Geometry check sheet. Reference: the model listing, model coordinates, mm. A direction names the side the tool comes from. Round coordinates to 2 decimals unless told otherwise and drop trailing zeros. Loops run counter-clockwise (first coordinate to the right, second up) from the corner with the lowest first, then second, coordinate; pieces in that order, holes last. Notation, with made-up numbers: M 18.5,81.5 L 48.5,81.5 A31 cw 48.5,110.5 Z; hole C 59,-25 d9. An arc over 180 degrees is marked long. Use one line per item in the form item = value. Start each with the question number.
1. Go/stop test with flat-tipped pins: pin 1 (4 mm diameter, centred on y = -23.79, z = 7.45, fed in from +X); pin 2 (4 mm diameter, centred on x = 9.5, z = 4, fed in from -Y); pin 3 (2.5 mm diameter, centred on x = 7, z = 5.5, fed in from +Y). Record where each tip stops, or that it passes through.
2. Cross-section at D-D (x = -14.5). Record the boundary of the cut face in (y, z), then the cut area to 3 significant figures.
3. Cross-section at C-C (y = -14). Record the boundary of the cut face in (x, z).
4. Material ranges on line 1 (Y direction, x = -41.95, z = 7.45); line 2 (Y direction, x = -34, z = 9); line 3 (Y direction, x = -39.55, z = 7.45), recorded low to high.
5. Cross-section at B-B (z = 7.45). State how many separate pieces and enclosed holes the cut face has, then the cut area to 3 significant figures.
6. Set-up check for faces 4 (the flat face through (10.19, 5, 6)), 5 (the cylindrical face through (-40.73, -20.62, 7.03)), 6 (the cylindrical face through (9.75, -7.07, 5.92)): record each of +Z, -Z, +X, -X, +Y, -Y from which the full face is reachable in a straight line by a thin tool's end or side.
7. Cross-section at A-A (y = 0). Record the boundary of the cut face in (x, z).
8. Draft check along Y on faces 1 (the cylindrical face through (-41.796, -35.377, 6.084)), 2 (the flat face through (7.28, 5.25, 5.92)), 3 (the flat face through (-5, -10.19, 6)). Enter one of: pulls with the +Y half, pulls with the -Y half, needs draft (parallel to the pull), parting line crosses it, or undercut.
```python
from build123d import *

# Parameters (mm, degrees)
BOSS_EXTRUDE1_DEPTH = 12
FILLET1_R           = 5
FILLET2_R           = 5
CUT_EXTRUDE1_REACH  = 74.499
SKETCH3_R           = 3.2
CHAMFER1_SIZE       = 0.2


with BuildPart() as part:
    # Sketch2 → Boss-Extrude1 (new body)
    with BuildSketch(Plane.XY):
        with BuildLine():
            Line((-10.5918, -13), (-5.317126718, -13))
            Line((-5.317126718, -13), (-4.287512407, -13))
            ThreePointArc((-4.287512407, -13), (-3.333616586, -12.604883414), (-2.9385, -11.650987593))
            Line((-2.9385, -11.650987593), (-2.9385, -11.539212407))
            ThreePointArc((-2.9385, -11.539212407), (-3.333616586, -10.585316586), (-4.287512407, -10.1902))
            Line((-4.287512407, -10.1902), (-6.416408329, -10.1902))
            ThreePointArc((-6.416408329, -10.1902), (-7.137514675, -9.708134418), (-6.967711912, -8.857517813))
            Line((-6.967711912, -8.857517813), (-3.740331666, -5.636015806))
            ThreePointArc((-3.740331666, -5.636015806), (-2.808257752, -5.01414519), (-1.709253557, -4.7958))
            Line((-1.709253557, -4.7958), (1.709253557, -4.7958))
            ThreePointArc((1.709253557, -4.7958), (2.808257752, -5.01414519), (3.740331666, -5.636015806))
            Line((3.740331666, -5.636015806), (6.967711912, -8.857517813))
            ThreePointArc((6.967711912, -8.857517813), (7.137514675, -9.708134418), (6.416408329, -10.1902))
            Line((6.416408329, -10.1902), (4.287512407, -10.1902))
            ThreePointArc((4.287512407, -10.1902), (3.333616586, -10.585316586), (2.9385, -11.539212407))
            Line((2.9385, -11.539212407), (2.9385, -11.650987593))
            ThreePointArc((2.9385, -11.650987593), (3.333616586, -12.604883414), (4.287512407, -13))
            Line((4.287512407, -13), (5.317126718, -13))
            Line((5.317126718, -13), (9.550465633, -13))
            Line((9.550465633, -13), (10.564722121, -12.999847763))
            ThreePointArc((10.564722121, -12.999847763), (12.294654751, -12.29465435), (12.999847757, -10.564721553))
            Line((12.999847757, -10.564721553), (13, -9.550422515))
            Line((13, -9.550422515), (13, -6.3330836))
            Line((13, -6.3330836), (13, -5.3170836))
            Line((13, -5.3170836), (13, -4.287469289))
            ThreePointArc((13, -4.287469289), (12.604883414, -3.333573468), (11.650987593, -2.938456882))
            Line((11.650987593, -2.938456882), (11.539212407, -2.938456882))
            ThreePointArc((11.539212407, -2.938456882), (10.585316586, -3.333573468), (10.1902, -4.287469289))
            Line((10.1902, -4.287469289), (10.1902, -6.402089023))
            ThreePointArc((10.1902, -6.402089023), (9.74154152, -7.073969797), (8.94902056, -6.917034355))
            Line((8.94902056, -6.917034355), (5.652895046, -3.628441884))
            ThreePointArc((5.652895046, -3.628441884), (5.027976112, -2.694919539), (4.8085, -1.593185507))
            Line((4.8085, -1.593185507), (4.8085, 1.593185507))
            ThreePointArc((4.8085, 1.593185507), (5.027976112, 2.694919539), (5.652895046, 3.628441884))
            Line((5.652895046, 3.628441884), (8.94902056, 6.917034355))
            ThreePointArc((8.94902056, 6.917034355), (9.74154152, 7.073969797), (10.1902, 6.402089023))
            Line((10.1902, 6.402089023), (10.1902, 4.287469289))
            ThreePointArc((10.1902, 4.287469289), (10.585316586, 3.333573468), (11.539212407, 2.938456882))
            Line((11.539212407, 2.938456882), (11.650987593, 2.938456882))
            ThreePointArc((11.650987593, 2.938456882), (12.604883414, 3.333573468), (13, 4.287469289))
            Line((13, 4.287469289), (13, 5.3170836))
            Line((13, 5.3170836), (13, 6.3330836))
            Line((13, 6.3330836), (13, 9.550422515))
            Line((13, 9.550422515), (18, 9.550422515))
            Line((18, 9.550422515), (18, -25))
            Line((18, -25), (0, -25))
            Line((0, -25), (0, -36.8026666))
            Line((0, -36.8026666), (-12, -36.8026666))
            Line((-12, -36.8026666), (-43.3, -36.8026666))
            Line((-43.3, -36.8026666), (-43.3, -31.8026666))
            Line((-43.3, -31.8026666), (-43.3, 6.7473334))
            Line((-43.3, 6.7473334), (-28.3, 6.7473334))
            Line((-28.3, 6.7473334), (-28.3, 1.7473334))
            Line((-28.3, 1.7473334), (-38.3, 1.7473334))
            Line((-38.3, 1.7473334), (-38.3, -31.8026666))
            Line((-38.3, -31.8026666), (-12.3, -31.8026666))
            Line((-12.3, -31.8026666), (-12.3, -13))
            Line((-12.3, -13), (-10.5918, -13))
        make_face()
    extrude(amount=BOSS_EXTRUDE1_DEPTH)

    # Fillet1
    fillet1_edges = [part.edges().sort_by_distance(p)[0] for p in [
        (0, -36.8026666, 6),
        (18, -25, 6),
        (0, -25, 6),
    ]]
    fillet(fillet1_edges, radius=FILLET1_R)

    # Fillet2
    fillet2_edges = [part.edges().sort_by_distance(p)[0] for p in [
        (-43.3, -36.8026666, 6),
        (-43.3, 6.7473334, 6),
    ]]
    fillet(fillet2_edges, radius=FILLET2_R)

    # Sketch3 → Cut-Extrude1 (cut, up to next)
    with BuildSketch(Plane.ZY.offset(43.3), mode=Mode.PRIVATE) as cut_extrude1_sk1:
        with Locations((7.45, -23.7926666)):
            Circle(SKETCH3_R)
    cut_extrude1_tool1 = extrude(cut_extrude1_sk1.sketch, amount=-CUT_EXTRUDE1_REACH, mode=Mode.PRIVATE) & part.part
    # Sketch3 → Cut-Extrude1 (cut, up to next)
    with BuildSketch(Plane.ZY.offset(43.3), mode=Mode.PRIVATE) as cut_extrude1_sk2:
        with Locations((7.45, -4.5926666)):
            Circle(SKETCH3_R)
    cut_extrude1_tool2 = extrude(cut_extrude1_sk2.sketch, amount=-CUT_EXTRUDE1_REACH, mode=Mode.PRIVATE) & part.part
    add(cut_extrude1_tool1.solids().sort_by_distance((-43.3, -23.792667, 7.45))[0], mode=Mode.SUBTRACT)
    add(cut_extrude1_tool2.solids().sort_by_distance((-43.3, -4.592667, 7.45))[0], mode=Mode.SUBTRACT)

    # Chamfer1
    chamfer1_edges = [part.edges().sort_by_distance(p)[0] for p in [
        (-43.3, -23.7926666, 4.25),
        (-43.3, -4.5926666, 4.25),
    ]]
    chamfer(chamfer1_edges, length=CHAMFER1_SIZE)


solid = part.part
```
Reported:
q1.pin_1 = 17.67
q1.pin_2 = -25
q1.pin_3 = 6.22
q2.outline = M -36.8,0 L -31.8,0 L -31.8,12 L -36.8,12 Z
q2.area = 60.0 mm²
q3.outline = M -43.3,0 L -38.3,0 L -38.3,12 L -43.3,12 Z; M -12.3,0 L 18,0 L 18,12 L -12.3,12 Z
q4.line_1 = -35.22 to -26.99, -20.59 to -7.79, -1.39 to 5.16
q4.line_2 = -36.8 to -31.8, 1.75 to 6.75
q4.line_3 = -36.64 to -26.99, -20.59 to -7.79, -1.39 to 6.59
q5.separate_pieces = 3
q5.enclosed_holes = 0
q5.area = 1,090 mm²
q6.face_4 = +Z, -Z, +Y
q6.face_5 = -X
q6.face_6 = +Z, -Z
q7.outline = M -43.3,0 L -38.3,0 L -38.3,12 L -43.3,12 Z; M 4.81,0 L 18,0 L 18,12 L 4.81,12 Z
q8.face_1 = pulls with the -Y half
q8.face_2 = pulls with the +Y half
q8.face_3 = undercut
